from build123d import *

# Parameters (mm, degrees)
BOSS_EXTRUDE1_DEPTH = 200
SKETCH5_R           = 1.5
CUT_EXTRUDE2_DEPTH  = 9
SKETCH6_R           = 1
CUT_EXTRUDE3_DEPTH  = 7
SKETCH7_R           = 1
CUT_EXTRUDE4_DEPTH  = 7


with BuildPart() as part:
    # Sketch1 → Boss-Extrude1 (new body)
    with BuildSketch(Plane.XY):
        with BuildLine():
            Line((-40, 31.315172042), (-40, 29.209945224))
            ThreePointArc((-40, 29.209945224), (0, 49.53), (40, 29.209945224))
            Line((40, 29.209945224), (40, 31.315172042))
            ThreePointArc((40, 31.315172042), (0, 50.8), (-40, 31.315172042))
        make_face()
    extrude(amount=BOSS_EXTRUDE1_DEPTH)

    # Sketch5 → Cut-Extrude2 (cut)
    with BuildSketch(Plane(origin=(-693.222728567, -633.307165687, 0), x_dir=(0.698885638, 0.715233434, 0), z_dir=(-0.715233434, 0.698885638, 0))):
        with Locations((937.445867756, -30)):
            Circle(SKETCH5_R)
        with Locations((937.445867756, -55.4)):
            Circle(SKETCH5_R)
        with Locations((937.445867756, -144.6)):
            Circle(SKETCH5_R)
        with Locations((937.445867756, -170)):
            Circle(SKETCH5_R)
    extrude(amount=-CUT_EXTRUDE2_DEPTH, mode=Mode.SUBTRACT)

    # Sketch6 → Cut-Extrude3 (cut)
    with BuildSketch(Plane(origin=(24.145050499, 41.582102129, -52.4), x_dir=(0, 0, 1), z_dir=(-0.502144913, -0.864783491, 0))):
        with Locations((247.4, 6)):
            Circle(SKETCH6_R)
        with Locations((247.4, -6)):
            Circle(SKETCH6_R)
        with Locations((57.4, 6)):
            Circle(SKETCH6_R)
        with Locations((57.4, -6)):
            Circle(SKETCH6_R)
    extrude(amount=-CUT_EXTRUDE3_DEPTH, mode=Mode.SUBTRACT)

    # Sketch7 → Cut-Extrude4 (cut)
    with BuildSketch(Plane(origin=(-24.145050502, 41.582102128, -52.4), x_dir=(0.864783491, 0.502144913, 0), z_dir=(0.502144913, -0.864783491, 0))):
        with Locations((-6, 247.4)):
            Circle(SKETCH7_R)
        with Locations((6, 247.4)):
            Circle(SKETCH7_R)
        with Locations((-6, 57.4)):
            Circle(SKETCH7_R)
        with Locations((6, 57.4)):
            Circle(SKETCH7_R)
    extrude(amount=-CUT_EXTRUDE4_DEPTH, mode=Mode.SUBTRACT)


solid = part.part
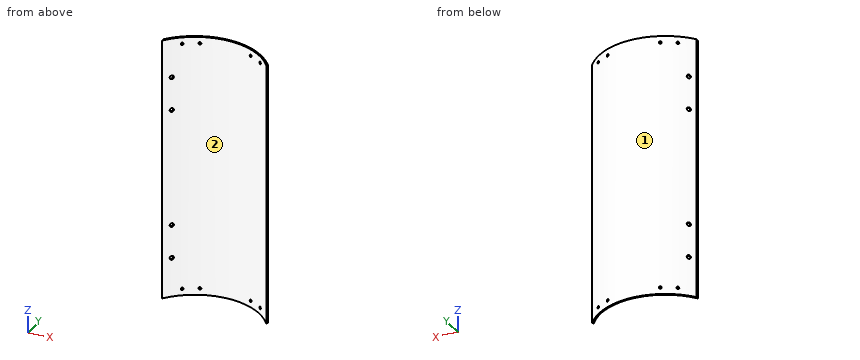
Design review of the part built by this model. Coordinates are the model's own, in mm. Face numbers are marked on the shaded views. Round coordinates to 2 decimals unless told otherwise and drop trailing zeros. Loops run counter-clockwise (first coordinate to the right, second up) from the corner with the lowest first, then second, coordinate; pieces in that order, holes last. Notation, with made-up numbers: (60.25, -1) - (114.25, -1) arc R27 cw to (114.25, 27) - close; hole circle Ø6 at (64, 63.25). An arc over 180 degrees is marked (long way). One line per item, written item: value. Start each with the question number.
1) Consider section A-A on z = 36.5. Give the boundary of the cut face in (x, y).
2) Consider section B-B on x = 7. Give the boundary of the cut face in (y, z).
3) To check wall thickness, follow L1, parallel to Z at x = -30, y = 40.25; L2, parallel to X at y = 38.25, z = 101.5; L3, parallel to X at y = 36.25, z = 122.5. State the ranges of each line that lie inside material, in increasing order. Write a range as from..to.
4) Insertion check: pin 1 Ø4 at (x, z) = (10.5, 120.5) entering from +Y; pin 2 Ø6 at (y, z) = (38.5, 90.5) entering from +X; pin 3 Ø5 at (y, z) = (38.5, 44) entering from -X; pin 4 Ø5 at (x, y) = (-29, 40.5) entering from -Z. Each pin has a flat end and moves straight along its axis. Give the tip position at first contact, or say it passes through.
5) Draft analysis for pull direction X (two halves, no side actions). For the marked faces 1 and 2, state which applies: +X half, -X half, draft (parallel to the pull), parting line (faces both ways), or undercut.
Reported:
1. outline: (-40, 29.21) arc R49.53 cw to (40, 29.21) - (40, 31.32) arc R50.8 ccw to (-40, 31.32) - close
2. outline: (49.03, 0) - (50.32, 0) - (50.32, 200) - (49.03, 200) - close
3. L1: z = 0..4.04, 5.96..194.04, 195.96..200
3. L2: x = -33.43..-31.47, 31.47..33.43
3. L3: x = -35.59..-33.75, 33.75..35.59
4. pin 1: stops at y = 50.08
4. pin 2: stops at x = 36.34
4. pin 3: stops at x = -35.84
4. pin 4: stops at z = 0
5. face 1: parting line
5. face 2: undercut
